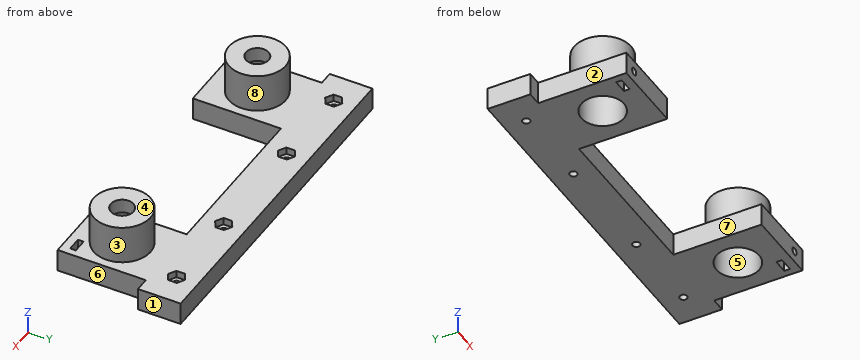
from build123d import *

# Parameters (mm, degrees)
SKETCH1_W               = 122
SKETCH1_H               = 15
BOSS_EXTRUDE1_DEPTH     = 8
SKETCH2_R               = 1.3
CUT_EXTRUDE1_DEPTH      = 1
CUT_EXTRUDE1_DEPTH_BACK = 9
CUT_EXTRUDE3_DEPTH      = 2.5
SKETCH5_W               = 26
SKETCH5_H               = 31
SKETCH5_R               = 7.5
BOSS_EXTRUDE2_DEPTH     = 8
SKETCH6_R               = 10
SKETCH6_R_2             = 7.5
BOSS_EXTRUDE3_DEPTH     = 8.5
SKETCH7_R               = 10
SKETCH7_R_2             = 4
BOSS_EXTRUDE4_DEPTH     = 5
SKETCH8_R               = 1.3
CUT_EXTRUDE4_DEPTH      = 5
SKETCH9_W               = 5
SKETCH9_H               = 2
CUT_EXTRUDE5_DEPTH      = 14.5
CUT_EXTRUDE5_DEPTH_BACK = 9


with BuildPart() as part:
    # Sketch1 → Boss-Extrude1 (new body)
    with BuildSketch(Plane.XY):
        Rectangle(SKETCH1_W, SKETCH1_H)
    extrude(amount=BOSS_EXTRUDE1_DEPTH)

    # Sketch2 → Cut-Extrude1 (cut, two sides)
    with BuildSketch(Plane.XY.offset(8)) as cut_extrude1_sk:
        with Locations((-20, 0)):
            Circle(SKETCH2_R)
        with Locations((20, 0)):
            Circle(SKETCH2_R)
        with Locations((-50, 0)):
            Circle(SKETCH2_R)
        with Locations((50, 0)):
            Circle(SKETCH2_R)
    extrude(amount=CUT_EXTRUDE1_DEPTH, mode=Mode.SUBTRACT)
    extrude(cut_extrude1_sk.sketch, amount=-CUT_EXTRUDE1_DEPTH_BACK, mode=Mode.SUBTRACT)

    # Sketch4 → Cut-Extrude3 (cut)
    with BuildSketch(Plane.XY.offset(8)):
        Polygon((-50, 3), (-52.598076211, 1.5), (-52.598076211, -1.5), (-50, -3), (-47.401923789, -1.5), (-47.401923789, 1.5), align=None)
        Polygon((-20, 3), (-22.598076211, 1.5), (-22.598076211, -1.5), (-20, -3), (-17.401923789, -1.5), (-17.401923789, 1.5), align=None)
        Polygon((20, 3), (17.401923789, 1.5), (17.401923789, -1.5), (20, -3), (22.598076211, -1.5), (22.598076211, 1.5), align=None)
        Polygon((50, 3), (47.401923789, 1.5), (47.401923789, -1.5), (50, -3), (52.598076211, -1.5), (52.598076211, 1.5), align=None)
    extrude(amount=-CUT_EXTRUDE3_DEPTH, mode=Mode.SUBTRACT)

    # Sketch5 → Boss-Extrude2 (add)
    with BuildSketch(Plane.XY):
        with Locations((-43, -23)):
            Rectangle(SKETCH5_W, SKETCH5_H)
        with Locations((-43, -23)):
            Circle(SKETCH5_R, mode=Mode.SUBTRACT)
        with Locations((43, -23)):
            Rectangle(SKETCH5_W, SKETCH5_H)
        with Locations((43, -23)):
            Circle(SKETCH5_R, mode=Mode.SUBTRACT)
    extrude(amount=BOSS_EXTRUDE2_DEPTH)

    # Sketch6 → Boss-Extrude3 (add)
    with BuildSketch(Plane.XY.offset(8)):
        with Locations((-43, -23)):
            Circle(SKETCH6_R)
        with Locations((-43, -23)):
            Circle(SKETCH6_R_2, mode=Mode.SUBTRACT)
        with Locations((43, -23)):
            Circle(SKETCH6_R)
        with Locations((43, -23)):
            Circle(SKETCH6_R_2, mode=Mode.SUBTRACT)
    extrude(amount=BOSS_EXTRUDE3_DEPTH)

    # Sketch7 → Boss-Extrude4 (add)
    with BuildSketch(Plane.XY.offset(16.5)):
        with Locations((-43, -23)):
            Circle(SKETCH7_R)
        with Locations((-43, -23)):
            Circle(SKETCH7_R_2, mode=Mode.SUBTRACT)
        with Locations((43, -23)):
            Circle(SKETCH7_R)
        with Locations((43, -23)):
            Circle(SKETCH7_R_2, mode=Mode.SUBTRACT)
    extrude(amount=BOSS_EXTRUDE4_DEPTH)

    # Sketch8 → Cut-Extrude4 (cut)
    with BuildSketch(Plane.XZ.offset(38.5)):
        with Locations((51, 4)):
            Circle(SKETCH8_R)
        with Locations((-51, 4)):
            Circle(SKETCH8_R)
    extrude(amount=-CUT_EXTRUDE4_DEPTH, mode=Mode.SUBTRACT)

    # Sketch9 → Cut-Extrude5 (cut, two sides)
    with BuildSketch(Plane.XY.offset(8)) as cut_extrude5_sk:
        with Locations((-51, -34.5)):
            Rectangle(SKETCH9_W, SKETCH9_H)
        with Locations((51, -34.5)):
            Rectangle(SKETCH9_W, SKETCH9_H)
    extrude(amount=CUT_EXTRUDE5_DEPTH, mode=Mode.SUBTRACT)
    extrude(cut_extrude5_sk.sketch, amount=-CUT_EXTRUDE5_DEPTH_BACK, mode=Mode.SUBTRACT)


solid = part.part
Geometry check sheet. Reference: the model listing, model coordinates, mm. Face numbers are marked on the shaded views. A direction names the side the tool comes from. Round coordinates to 2 decimals unless told otherwise and drop trailing zeros. Loops run counter-clockwise (first coordinate to the right, second up) from the corner with the lowest first, then second, coordinate; pieces in that order, holes last. Notation, with made-up numbers: (31.25, 80) -> (56.25, 80) arc R22 ccw to (56.25, 111) -> close; hole circle Ø8 at (23.25, -3). An arc over 180 degrees is marked (long way). Answer as a JSON object with one key per item and string values. Group by question number.
Item 1: Cross-section at C-C, the plane y = -17.5. Record the cut outline in (x, z), plus the area to 3 significant figures.
Item 2: Set-up check for the marked faces 4, 5, 6, 7 and 8: record each of +Z, -Z, +X, -X, +Y, -Y from which the full face is reachable in a straight line by a thin tool's end or side.
Item 3: Cross-section at A-A, the plane z = 19.25. Record the cut outline in (x, y), plus the area to 3 significant figures.
Item 4: Depth check by flat-ended pin: pin 1 Ø6 at (y, z) = (-25, 7.5) entering from -X; pin 2 Ø6 at (y, z) = (-21, 15) entering from +X; pin 3 Ø0.6 at (y, z) = (-34.5, 6) entering from +X; pin 4 Ø2 at (x, y) = (-50, 0) entering from +Z. Enter the tip coordinate at first touch or a pass-through.
Item 5: Cross-section at B-B, the plane x = 43. Record the cut outline in (y, z), plus the area to 4 significant figures.
Item 6: Cross-section at D-D, the plane y = 0. Count the separate pieces of the cut face and the enclosed holes in it, plus the area to 3 significant figures.
Item 7: Thickness scan on line 1 along Y through (x, z) = (43, 4.75); line 2 along Z through (x, y) = (-51, -36.2); line 3 along X through (y, z) = (0.5, 3.75). Record the ranges inside material, lowest first.
Item 8: Release check for a two-part mould opening along X. For the marked faces 1, 2 and 3 record: pulls with the +X half, pulls with the -X half, needs draft (parallel to the pull), parting line crosses it, or undercut.
Determined:
{
 "1": {"outline": "(-56, 0) -> (-48.1, 0) -> (-48.1, 16.5) -> (-37.9, 16.5) -> (-37.9, 0) -> (-30, 0) -> (-30, 8) -> (-34.65, 8) -> (-34.65, 21.5) -> (-51.35, 21.5) -> (-51.35, 8) -> (-56, 8) -> close; (30, 0) -> (37.9, 0) -> (37.9, 16.5) -> (48.1, 16.5) -> (48.1, 0) -> (56, 0) -> (56, 8) -> (51.35, 8) -> (51.35, 21.5) -> (34.65, 21.5) -> (34.65, 8) -> (30, 8) -> close", "area": "530 mm²"},
 "2": {"face 4": "+Z, +X, -X, +Y, -Y", "face 5": "-Z", "face 6": "+Z, -Z, +X, -Y", "face 7": "+Z, -Z, -Y", "face 8": "+Z"},
 "3": {"outline": "circle Ø20 at (-43, -23); circle Ø20 at (43, -23); hole circle Ø8 at (-43, -23); hole circle Ø8 at (43, -23)", "area": "528 mm²"},
 "4": {"pin 1": "stops at x = -56", "pin 2": "stops at x = 53", "pin 3": "stops at x = 56", "pin 4": "passes through"},
 "5": {"outline": "(-38.5, 0) -> (-30.5, 0) -> (-30.5, 16.5) -> (-27, 16.5) -> (-27, 21.5) -> (-33, 21.5) -> (-33, 8) -> (-38.5, 8) -> close; (-19, 16.5) -> (-15.5, 16.5) -> (-15.5, 0) -> (7.5, 0) -> (7.5, 8) -> (-13, 8) -> (-13, 21.5) -> (-19, 21.5) -> close", "area": "350.5 mm²"},
 "6": {"separate pieces": "5", "enclosed holes": "0", "area": "867 mm²"},
 "7": {"line 1": "y = -38.5 to -30.5, -15.5 to 7.5", "line 2": "z = 0 to 2.7, 5.3 to 8", "line 3": "x = -61 to -51.2, -48.8 to -21.2, -18.8 to 18.8, 21.2 to 48.8, 51.2 to 61"},
 "8": {"face 1": "pulls with the +X half", "face 2": "pulls with the -X half", "face 3": "undercut"}
}
